Could you check a few things on this model? Use its own coordinates, in mm. A direction names the side the tool comes from. Give positions to 0.01 mm unless a question says otherwise; leave off trailing zeros. Order: outer loops, then holes, each group sorted by start corner. A loop starts at its lowest first (then second) coordinate and runs counter-clockwise, first axis right, second up. Notation, with made-up numbers: M -39,1.5 L 16,1.5 A19 cw 16,28.5 Z; hole C -12.75,65.5 d2. An arc over 180 degrees is marked long. Return JSON: item names as keys, results as strings. Group by question number.
```python
from build123d import *

# Parameters (mm, degrees)
ESQUISSE2_R                  = 70
ESQUISSE2_R_2                = 20
BOSS_EXTRU_1_DEPTH           = 140
ENL_V_MAT_EXTRU_1_DEPTH      = 172.464281995
ENL_V_MAT_EXTRU_1_DEPTH_BACK = 172.464281995
ESQUISSE3_W                  = 15
ESQUISSE3_H                  = 70
ESQUISSE7_W                  = 155
ESQUISSE7_H                  = 70
BOSS_EXTRU_3_DEPTH           = 70
ENL_V_MAT_EXTRU_5_DEPTH      = 206.304651676
ENL_V_MAT_EXTRU_5_DEPTH_BACK = 206.304651676
ESQUISSE11_W                 = 50
ESQUISSE11_H                 = 80
ESQUISSE10_R                 = 20
ENL_V_MAT_EXTRU_4_DEPTH      = 180


with BuildPart() as part:
    # Esquisse2 → Boss.-Extru.1 (new body)
    with BuildSketch(Plane(origin=(0, 0, 0), x_dir=(1, 0, 0), z_dir=(0, 1, 0))):
        with Locations(Location((0, 0, 0), (0, 0, 270))):
            Circle(ESQUISSE2_R)
        with Locations(Location((0, 0, 0), (0, 0, 270))):
            Circle(ESQUISSE2_R_2, mode=Mode.SUBTRACT)
    extrude(amount=BOSS_EXTRU_1_DEPTH)

    # Esquisse3 → Enlèv. mat.-Extru.1 (cut, two sides: drawn at the far end of the back side and taken through both)
    with BuildSketch(Plane(origin=(0, 0, 0), x_dir=(0, 0, -1), z_dir=(1, 0, 0)).offset(-ENL_V_MAT_EXTRU_1_DEPTH_BACK)):
        Rectangle(ESQUISSE3_W, ESQUISSE3_H)
    extrude(amount=ENL_V_MAT_EXTRU_1_DEPTH + ENL_V_MAT_EXTRU_1_DEPTH_BACK, mode=Mode.SUBTRACT)

    # Esquisse7 → Boss.-Extru.3 (add, symmetric)
    with BuildSketch(Plane(origin=(0, 0, 0), x_dir=(0, 0, -1), z_dir=(1, 0, 0))):
        with Locations((-77.5, 80)):
            Rectangle(ESQUISSE7_W, ESQUISSE7_H)
    extrude(amount=BOSS_EXTRU_3_DEPTH, both=True)

    # Esquisse11 → Enlèv. mat.-Extru.5 (cut, two sides: drawn at the far end of the back side and taken through both)
    with BuildSketch(Plane(origin=(0, 115, 0), x_dir=(1, 0, 0), z_dir=(0, 1, 0)).offset(-ENL_V_MAT_EXTRU_5_DEPTH_BACK)):
        with Locations((0, -155)):
            Rectangle(ESQUISSE11_W, ESQUISSE11_H)
    extrude(amount=ENL_V_MAT_EXTRU_5_DEPTH + ENL_V_MAT_EXTRU_5_DEPTH_BACK, mode=Mode.SUBTRACT)

    # Esquisse10 → Enlèv. mat.-Extru.4 (cut, symmetric)
    with BuildSketch(Plane(origin=(0, 140, 0), x_dir=(1, 0, 0), z_dir=(0, 1, 0))):
        with Locations(Location((0, 0, 0), (0, 0, 22.024312837))):
            Circle(ESQUISSE10_R)
    extrude(amount=ENL_V_MAT_EXTRU_4_DEPTH, both=True, mode=Mode.SUBTRACT)


solid = part.part
```
1. Imagine slicing it at B-B, the plane y = 74.5. Please give me the cut outline in (x, z), plus the area to 3 significant figures.
2. For pin 1 (17.5 mm diameter, centred on x = -33.5, y = 20, fed in from +Z); pin 2 (12 mm diameter, centred on x = 39.5, z = 80.5, fed in from -Y); pin 3 (10 mm diameter, centred on y = 42.5, z = 27.5, fed in from -X); pin 4 (1.5 mm diameter, centred on x = 18.5, y = 75.5, fed in from +Z), each with a flat end and sliding along its axis, tell me the tip position at first contact or that it passes through.
3. Imagine slicing it at C-C, the plane x = 0. Please give me the cut outline in (y, z).
4. Which directions (+Z, -Z, +X, -X, +Y, -Y) give clear straight access to the entire face, cutting with the end or side of a thin tool? Please do faces 4 (the flat face through (-25, 80, 135)), 5 (the cylindrical face through (3.078, 69.02, -69.932)), 6 (the flat face through (-47, 80, 155)), 7 (the flat face through (44, 17, 7.5)).
5. I need wall thicknesses on L1, parallel to X at y = 59.5, z = 0; L2, parallel to Y at x = -50, z = 51.5; L3, parallel to Z at x = 62, y = 33. Which ranges of each line are inside material? Lowest first, please. Write a range as from..to.
6. Imagine slicing it at A-A, the plane z = 120. Please give me the cut outline in (x, y).
7. Imagine slicing it at D-D, the plane x = 43. Please give me the cut outline in (y, z).
8. If we mould it in two halves opening along X, with no side actions, what happens to faces 1 (the flat face through (0, 80, 115)), 2 (the flat face through (-70, 80, 79)), 3 (the flat face through (1, 45, 96))? For each: pulls with the +X half, pulls with the -X half, needs draft (parallel to the pull), parting line crosses it, or undercut.
Values:
{
 "1": {"outline": "M -70,0 A70 ccw 70,0 L 70,155 L 25,155 L 25,115 L -25,115 L -25,155 L -70,155 Z; hole C 0,0 d40", "area": "26,100 mm²"},
 "2": {"pin 1": "stops at z = 65.48", "pin 2": "stops at y = 45", "pin 3": "stops at x = -70", "pin 4": "stops at z = 115"},
 "3": {"outline": "M 0,-70 L 140,-70 L 140,-20 L 0,-20 Z; M 0,20 L 140,20 L 140,70 L 115,70 L 115,115 L 45,115 L 45,70 L 0,70 Z"},
 "4": {"face 4": "+Z, +Y, -Y", "face 5": "none", "face 6": "+Z, +X, -X, +Y, -Y", "face 7": "+X, -X, -Y"},
 "5": {"L1": "x = -70..-20, 20..70", "L2": "y = 45..115", "L3": "z = -32.5..-7.5, 7.5..32.5"},
 "6": {"outline": "M -70,45 L -25,45 L -25,115 L -70,115 Z; M 25,45 L 70,45 L 70,115 L 25,115 Z"},
 "7": {"outline": "M 0,-55.24 L 140,-55.24 L 140,55.24 L 115,55.24 L 115,155 L 45,155 L 45,55.24 L 0,55.24 L 0,7.5 L 35,7.5 L 35,-7.5 L 0,-7.5 Z"},
 "8": {"face 1": "undercut", "face 2": "pulls with the -X half", "face 3": "needs draft"}
}
